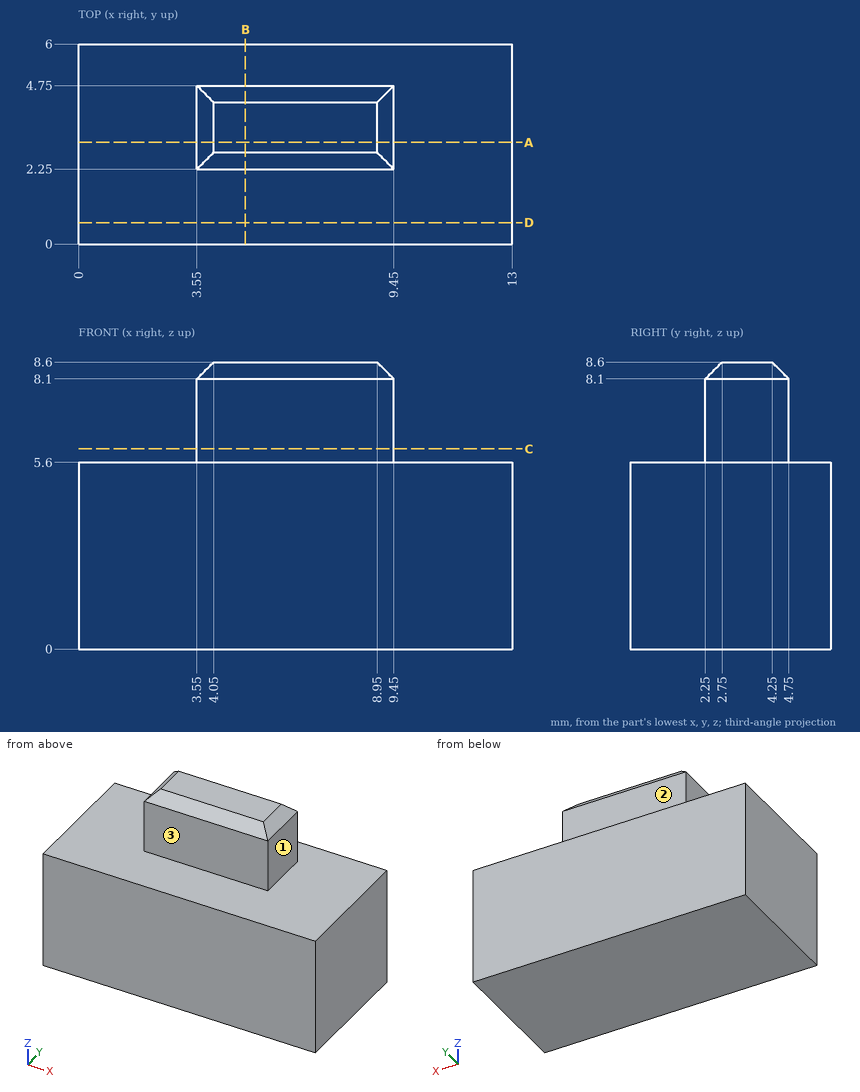
Print and shaded views of the part. All mm, measured from the part's lowest x, y and z. A direction names the side the tool comes from. Give positions to 0.01 mm unless a question says otherwise; leave off trailing zeros. Write each loop counter-clockwise with the first axis right and the second up, starting at its lowest first coordinate (ties: lowest second). Pieces come first, ordered by that corner, then holes. Notation, with made-up numbers: (-37, 35) - (-17, 35) arc R16 cw to (-17, 66) - close; hole circle Ø9 at (1.5, 73). An arc over 180 degrees is marked (long way). One line per question, with ' | ' between items. Start each with the question number.
(1) Slice it at B-B on x = 5. Write the cut outline in (y, z).
(2) Slice it at A-A on y = 3.05. Write the cut outline in (x, z), plus the area to 4 significant figures.
(3) Slice it at C-C on z = 6. Write the cut outline in (x, y), plus the area to 4 significant figures.
(4) Wall check: line 1 along Z through (x, y) = (1, 1.6); line 2 along X through (y, z) = (4.25, 5.75); line 3 along Y through (x, z) = (9, 7.5). Give the ranges that are in metal, low to high. Write a range as from..to.
(5) 3-axis set-ups, long thin cutter, end or side, ignore diameter. For the marked faces 1, 2 and 3: which of +Z, -Z, +X, -X, +Y, -Y reach the whole face in a straight line?
(6) Slice it at D-D on y = 0.65. Write the cut outline in (x, z), plus the area to 3 significant figures.
(7) Pin check, flat tips, straight feed: P1, Ø0.8, axis at y = 4, z = 7, coming from the -X side; P2, Ø0.8, axis at y = 4, z = 7, coming from the +X side; P3, Ø2, axis at x = 4.5, z = 7.5, coming from the -Y side; P4, Ø5, axis at x = 8.5, z = 4, coming from the -Y side. Stop position of each tip, or through.
Results below:
1) outline: (0, 0) - (6, 0) - (6, 5.6) - (4.75, 5.6) - (4.75, 8.1) - (4.25, 8.6) - (2.75, 8.6) - (2.25, 8.1) - (2.25, 5.6) - (0, 5.6) - close
2) outline: (0, 0) - (13, 0) - (13, 5.6) - (9.45, 5.6) - (9.45, 8.1) - (8.95, 8.6) - (4.05, 8.6) - (3.55, 8.1) - (3.55, 5.6) - (0, 5.6) - close | area: 90.25 mm^2
3) outline: (3.55, 2.25) - (9.45, 2.25) - (9.45, 4.75) - (3.55, 4.75) - close | area: 14.75 mm^2
4) line 1: 0..5.6 | line 2: 3.55..9.45 | line 3: 2.25..4.75
5) face 1: +Z, +X, +Y, -Y | face 2: +Z, +X, -X, +Y | face 3: +Z, +X, -X, -Y
6) outline: (0, 0) - (13, 0) - (13, 5.6) - (0, 5.6) - close | area: 72.8 mm^2
7) P1: x = 3.55 | P2: x = 9.45 | P3: y = 2.25 | P4: y = 0
